For this review, use the dimensioned drawing (mm, ordinates from the lowest corner) and the shaded views. A direction names the side the tool comes from. Give positions to 0.01 mm unless a question says otherwise; leave off trailing zeros. Order: outer loops, then holes, each group sorted by start corner. A loop starts at its lowest first (then second) coordinate and runs counter-clockwise, first axis right, second up.
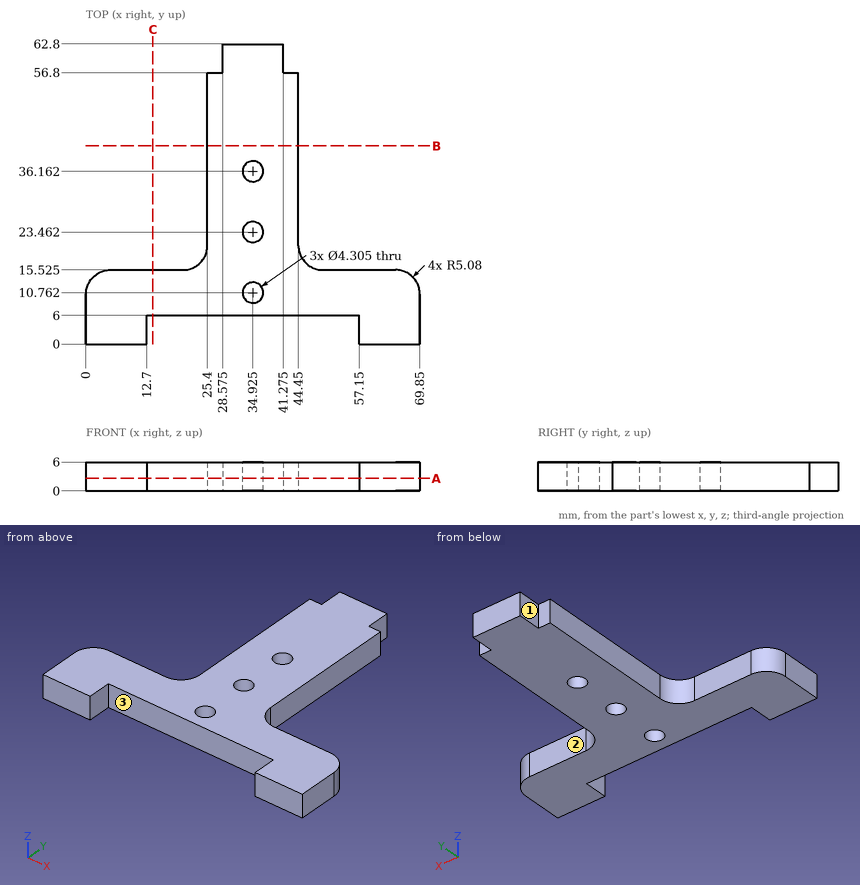
1. Take a section at C-C (x = 14). State the section outline as (y, z) points (1 decimal).
Recorded:
outline: (6, 0) - (15.5, 0) - (15.5, 6) - (6, 6) - close
2. Take a section at B-B (y = 41.5). State the section outline as (x, z) points.
Recorded:
outline: (25.4, 0) - (44.45, 0) - (44.45, 6) - (25.4, 6) - close
3. Machinability: for the marked faces 1, 2 and 3, which of the approach directions +Z, -Z, +X, -X, +Y, -Y give a long, thin tool a straight path to every point of the face, cutting with its end or side? Answer none if there is none.
Recorded:
face 1: +Z, -Z, -X, +Y
face 2: +Z, -Z, +X, +Y
face 3: +Z, -Z, -Y
4. Take a section at A-A (z = 2.6). State how many separate pieces and enclosed holes the cut face has, then the cut area to 3 significant figures.
Recorded:
separate pieces: 1
enclosed holes: 3
area: 1,640 mm2
5. For line 1 along Y through (x, z) = (53.5, 5.4) (1 decimal); line 2 along X through (y, z) = (33, 5.3); line 3 along X through (y, z) = (36, 2.05), list the stretches that pass through material, from the lowest coordinate up.
Recorded:
line 1: y = 6 to 15.5
line 2: x = 25.4 to 44.45
line 3: x = 25.4 to 32.78, 37.07 to 44.45
6. For pin 1 (7 mm diameter, centred on x = 34.92, y = 10.76, fed in from -Z); pin 2 (3 mm diameter, centred on y = 60, z = 1.5, fed in from +X) (1 decimal); pin 3 (1 mm diameter, centred on x = 42, z = 4, fed in from +Y); pin 4 (1.8 mm diameter, centred on y = 31, z = 3.5, fed in from -X), all flat-tipped, find the tip position at first contact; note any pin that passes through.
Recorded:
pin 1: stops at z = 0
pin 2: stops at x = 41.3
pin 3: stops at y = 56.8
pin 4: stops at x = 25.4
